```python
from build123d import *

# Parameters (mm, degrees)
M8_CLEARANCE_HOLE1_D     = 9.5758
M8_CLEARANCE_HOLE1_DEPTH = 7.239
M4_CLEARANCE_HOLE1_D     = 4.3688
M4_CLEARANCE_HOLE1_DEPTH = 7.239
M4_CLEARANCE_HOLE2_D     = 4.3688
M4_CLEARANCE_HOLE2_DEPTH = 7.239
CHAMFER1_SIZE            = 0.254
SKETCH8_R                = 8.600554372
BOSS_EXTRUDE1_DEPTH      = 21.717
SKETCH9_R                = 7.068084354
CUT_EXTRUDE1_DEPTH       = 29.956


with BuildPart() as part:
    # Sketch1 → Revolve1 (revolve)
    with BuildSketch(Plane(origin=(0, 0, 0), x_dir=(1, 0, 0), z_dir=(0, 1, 0))):
        with BuildLine():
            Line((16.891, 7.239), (0, 7.239))
            Line((0, 7.239), (0, 1.27))
            Line((0, 1.27), (5.321088826, 1.27))
            ThreePointArc((5.321088826, 1.27), (6.0579, 1.83769793), (6.794711174, 1.27))
            Line((6.794711174, 1.27), (9.144, 1.27))
            Line((9.144, 1.27), (9.144, 0.6604))
            Line((9.144, 0.6604), (10.7188, 1.233580325))
            Line((10.7188, 1.233580325), (10.7188, 0))
            Line((10.7188, 0), (16.891, 0))
            Line((16.891, 0), (16.891, 7.239))
        make_face()
    revolve(axis=Axis((0, 0, -7.239), (0, 0, 1)))

    # M8 Clearance Hole1
    with Locations(Plane(origin=(0, 0, -7.239), x_dir=(-1, 0, 0), z_dir=(0, 0, -1))):
        with Locations((0, 0)):
            Hole(M8_CLEARANCE_HOLE1_D / 2, depth=M8_CLEARANCE_HOLE1_DEPTH)

    # M4 Clearance Hole1
    with Locations(Plane.XY):
        with Locations((11.680431031, 6.7437), (0, -13.4874), (-11.680431031, -6.7437), (-11.680431031, 6.7437)):
            Hole(M4_CLEARANCE_HOLE1_D / 2, depth=M4_CLEARANCE_HOLE1_DEPTH)

    # M4 Clearance Hole2
    with Locations(Plane(origin=(0, 0, -7.239), x_dir=(-1, 0, 0), z_dir=(0, 0, -1))):
        with Locations((0, 13.4874), (-11.680431031, -6.7437)):
            Hole(M4_CLEARANCE_HOLE2_D / 2, depth=M4_CLEARANCE_HOLE2_DEPTH)

    # Chamfer1
    chamfer1_edges = [part.edges().sort_by_distance(p)[0] for p in [
        (-16.891, 0, 0),
        (-9.496031031, 6.7437, 0),
        (-9.496031031, 6.7437, -7.239),
        (-9.496031031, -6.7437, 0),
        (-9.496031031, -6.7437, -7.239),
        (2.1844, -13.4874, 0),
        (2.1844, -13.4874, -7.239),
        (13.864831031, 6.7437, 0),
        (13.864831031, 6.7437, -7.239),
        (9.496031031, -6.7437, -7.239),
        (9.496031031, -6.7437, 0),
        (-2.1844, 13.4874, -7.239),
        (-2.1844, 13.4874, 0),
        (-16.891, 0, -7.239),
    ]]
    chamfer(chamfer1_edges, length=CHAMFER1_SIZE)

    # Sketch8 → Boss-Extrude1 (add)
    with BuildSketch(Plane(origin=(0, 0, -7.239), x_dir=(-1, 0, 0), z_dir=(0, 0, -1))):
        Circle(SKETCH8_R)
    extrude(amount=BOSS_EXTRUDE1_DEPTH)

    # Sketch9 → Cut-Extrude1 (cut, through all)
    with BuildSketch(Plane(origin=(0, 0, -28.956), x_dir=(-1, 0, 0), z_dir=(0, 0, -1))):
        Circle(SKETCH9_R)
    extrude(amount=-CUT_EXTRUDE1_DEPTH, mode=Mode.SUBTRACT)


solid = part.part
```
Design review of the part built by this model. Coordinates are the model's own, in mm. A direction names the side the tool comes from. Give positions to 0.01 mm unless a question says otherwise; leave off trailing zeros. Order: outer loops, then holes, each group sorted by start corner. A loop starts at its lowest first (then second) coordinate and runs counter-clockwise, first axis right, second up. Notation, with made-up numbers: (75.5, -22) - (131.5, -22) arc R16 cw to (131.5, 0) - close; hole circle Ø6 at (34, 84). An arc over 180 degrees is marked (long way). Use a Markdown table: item, result. Add a question column.
(1) Mouldability with a two-part tool opening along Y and no side actions: class faces 3 (the face through (1.864, -8.396, -17.945)), 4 (the face through (-10.07, -5.27, -3.67)), 5 (the face through (9.597, 7.4, -3.667)), 6 (the face through (7, -7, -7.239)) as +Y half, -Y half, draft (parallel to the pull), parting line (faces both ways), or undercut.
(2) Clearance check with flat-ended pins moving along their axes: P1, Ø5, axis at x = 2.5, z = -24.5, coming from the +Y side; P2, Ø7, axis at x = 0, y = -13.49, coming from the -Z side; P3, Ø12, axis at y = 13, z = -21.5, coming from the +X side; P4, Ø4, axis at x = 11, z = -19, coming from the +Y side. State where each tip first meets the part, or that it passes through.
(3) Wall thickness on probe 1 along Y at (x, z) = (0, -2); probe 2 along X at (y, z) = (8, -2.25); probe 3 along Y at (x, z) = (0, -8): over which ranges is each line inside the solid? List them lowest first. Write a range as [from, to].
(4) Machinability: for faces 1 (the face through (10.07, -5.27, -3.57)), 2 (the face through (-10.71, 0.47, -0.61)), which of the approach directions +Z, -Z, +X, -X, +Y, -Y give a long, thin tool a straight path to every point of the face, cutting with its end or side? Answer none if there is none.
(5) Add section B-B on x = 0. Give the number of separate pieces and of enclosed holes in the cut face, then the cut area to 3 significant figures.
(6) Add section A-A on y = 0. Give the boundary of the cut face in (x, z) (3 decimals), then the cut area to 3 significant figures.
(7) Add section D-D on z = -20. Give the boundary of the cut face in (x, y).
(8) Add section C-C on z = -5.75. Give the boundary of the cut face in (x, y), then the cut area to 3 significant figures.
Report:
| question | item | result |
|---|---|---|
| 1 | face 3 | parting line |
| 1 | face 4 | undercut |
| 1 | face 5 | undercut |
| 1 | face 6 | draft |
| 2 | P1 | stops at y = 8.6 |
| 2 | P2 | stops at z = -7.24 |
| 2 | P3 | stops at x = 5 |
| 2 | P4 | passes through |
| 3 | probe 1 | y = [-16.89, -15.67], [-11.3, -7.07], [7.07, 11.3], [15.67, 16.89] |
| 3 | probe 2 | x = [-14.88, -13.47], [-9.89, 9.89], [13.47, 14.88] |
| 3 | probe 3 | y = [-8.6, -7.07], [7.07, 8.6] |
| 4 | face 1 | +Z, -Z |
| 4 | face 2 | +Z |
| 5 | separate pieces | 4 |
| 5 | enclosed holes | 0 |
| 5 | area | 137 mm² |
| 6 | outline | (-16.891, -6.985) - (-16.637, -7.239) - (-8.601, -7.239) - (-8.601, -28.956) - (-7.068, -28.956) - (-7.068, -1.27) - (-9.144, -1.27) - (-9.144, -0.66) - (-10.719, -1.234) - (-10.719, 0) - (-16.637, 0) - (-16.891, -0.254) - close; (7.068, -28.956) - (8.601, -28.956) - (8.601, -7.239) - (16.637, -7.239) - (16.891, -6.985) - (16.891, -0.254) - (16.637, 0) - (10.719, 0) - (10.719, -1.234) - (9.144, -0.66) - (9.144, -1.27) - (7.068, -1.27) - close |
| 6 | area | 200 mm² |
| 7 | outline | circle Ø17.2 at (0, 0); hole circle Ø14.14 at (0, 0) |
| 8 | outline | circle Ø33.78 at (0, 0); hole circle Ø4.37 at (-11.68, -6.74); hole circle Ø4.37 at (-11.68, 6.74); hole circle Ø14.14 at (0, 0); hole circle Ø4.37 at (0, -13.49); hole circle Ø4.37 at (0, 13.49); hole circle Ø4.37 at (11.68, -6.74); hole circle Ø4.37 at (11.68, 6.74) |
| 8 | area | 649 mm² |
